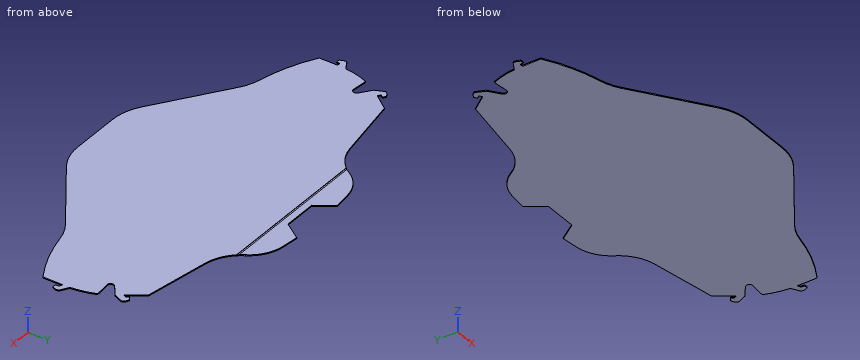
```python
from build123d import *

# Parameters (mm, degrees)
MAIN_SHAPE_DEPTH               = 0.6
TABS_DEPTH                     = 154.060061459
TABS_DEPTH_BACK                = 154.060061459
CHIN_GUARD_DEPTH               = 0.6
FILLET1_R                      = 30
QUICK_RELEASE_NOTCH_DEPTH      = 172.662513141
QUICK_RELEASE_NOTCH_DEPTH_BACK = 172.662513141
SKETCH8_W                      = 100
SKETCH8_H                      = 1
CUT_EXTRUDE3_DEPTH             = 0.2


with BuildPart() as part:
    # Sketch1 → Main Shape (new body)
    with BuildSketch(Plane.XY):
        with BuildLine():
            Line((-24, -91.764766734), (24, -91.764766734))
            Line((24, -91.764766734), (78.266232563, -84.05670244))
            ThreePointArc((78.266232563, -84.05670244), (97.655491519, -79.289252293), (115.711102551, -70.764766734))
            ThreePointArc((115.711102551, -70.764766734), (120.685143325, -65.658407438), (122.5, -58.764766734))
            ThreePointArc((122.5, -58.764766734), (120.227482046, -43.118277124), (113.597722286, -28.764766734))
            ThreePointArc((113.597722286, -28.764766734), (107.811505455, -22.955172168), (100.180351554, -19.955641477))
            Line((100.180351554, -19.955641477), (60.74391922, -13.264766734))
            ThreePointArc((60.74391922, -13.264766734), (50.804108255, -9.246591688), (43.461443341, -1.434367632))
            ThreePointArc((43.461443341, -1.434367632), (36.448172688, 5.805997675), (26.941855461, 9.15842781))
            Line((26.941855461, 9.15842781), (17, 10.235233266))
            Line((17, 10.235233266), (10, 0))
            Line((10, 0), (-10, 0))
            Line((-10, 0), (-17, 10.235233266))
            Line((-17, 10.235233266), (-26.941855461, 9.15842781))
            ThreePointArc((-26.941855461, 9.15842781), (-36.448172688, 5.805997675), (-43.461443341, -1.434367632))
            ThreePointArc((-43.461443341, -1.434367632), (-50.804108255, -9.246591688), (-60.74391922, -13.264766734))
            Line((-60.74391922, -13.264766734), (-100.180351554, -19.955641477))
            ThreePointArc((-100.180351554, -19.955641477), (-107.811505455, -22.955172168), (-113.597722286, -28.764766734))
            ThreePointArc((-113.597722286, -28.764766734), (-120.227482046, -43.118277124), (-122.5, -58.764766734))
            ThreePointArc((-122.5, -58.764766734), (-120.685143325, -65.658407438), (-115.711102551, -70.764766734))
            ThreePointArc((-115.711102551, -70.764766734), (-97.655491519, -79.289252293), (-78.266232563, -84.05670244))
            Line((-78.266232563, -84.05670244), (-24, -91.764766734))
        make_face()
    extrude(amount=MAIN_SHAPE_DEPTH)

    # Sketch2 → Tabs (cut, two sides: drawn at the far end of the back side and taken through both)
    with BuildSketch(Plane.XY.offset(0.6).offset(-TABS_DEPTH_BACK)):
        with BuildLine():
            Line((-121, -59.764766734), (-121, -57.764766734))
            Line((-121, -57.764766734), (-115.834995394, -54.767490128))
            ThreePointArc((-115.834995394, -54.767490128), (-113.511139955, -43.427720083), (-108.566362279, -32.961590783))
            Line((-108.566362279, -32.961590783), (-110.9, -27.464766734))
            Line((-110.9, -27.464766734), (-109.7, -25.864766734))
            Line((-109.7, -25.864766734), (-107.7, -24.864766734))
            Line((-107.7, -24.864766734), (-106.1, -26.064766734))
            Line((-106.1, -26.064766734), (-107.3, -27.664766734))
            Line((-107.3, -27.664766734), (-105.7, -28.864766734))
            Line((-105.7, -28.864766734), (-98.84870892, -19.729711961))
            Line((-98.84870892, -19.729711961), (-100.180351554, -19.955641477))
            ThreePointArc((-100.180351554, -19.955641477), (-107.811505455, -22.955172168), (-113.597722286, -28.764766734))
            ThreePointArc((-113.597722286, -28.764766734), (-120.227482046, -43.118277124), (-122.5, -58.764766734))
            ThreePointArc((-122.5, -58.764766734), (-120.767844146, -65.510135516), (-116, -70.586357152))
            Line((-116, -70.586357152), (-116, -59.764766734))
            Line((-116, -59.764766734), (-118, -59.764766734))
            Line((-118, -59.764766734), (-118, -61.764766734))
            Line((-118, -61.764766734), (-120, -61.764766734))
            Line((-120, -61.764766734), (-121, -59.764766734))
        make_face()
        with BuildLine():
            Line((109.7, -25.864766734), (110.9, -27.464766734))
            Line((110.9, -27.464766734), (108.566362279, -32.961590783))
            ThreePointArc((108.566362279, -32.961590783), (113.511139955, -43.427720083), (115.834995394, -54.767490128))
            Line((115.834995394, -54.767490128), (121, -57.764766734))
            Line((121, -57.764766734), (121, -59.764766734))
            Line((121, -59.764766734), (120, -61.764766734))
            Line((120, -61.764766734), (118, -61.764766734))
            Line((118, -61.764766734), (118, -59.764766734))
            Line((118, -59.764766734), (116, -58.764766734))
            Line((116, -58.764766734), (116, -70.586357152))
            ThreePointArc((116, -70.586357152), (120.767844146, -65.510135516), (122.5, -58.764766734))
            ThreePointArc((122.5, -58.764766734), (120.227482046, -43.118277124), (113.597722286, -28.764766734))
            ThreePointArc((113.597722286, -28.764766734), (107.811505455, -22.955172168), (100.180351554, -19.955641477))
            Line((100.180351554, -19.955641477), (98.84870892, -19.729711961))
            Line((98.84870892, -19.729711961), (105.979039493, -29.610311845))
            Line((105.979039493, -29.610311845), (106.979039493, -27.610311845))
            Line((106.979039493, -27.610311845), (105.920723622, -26.199224018))
            Line((105.920723622, -26.199224018), (107.7, -24.864766734))
            Line((107.7, -24.864766734), (109.7, -25.864766734))
        make_face()
    extrude(amount=TABS_DEPTH + TABS_DEPTH_BACK, mode=Mode.SUBTRACT)

    # Sketch5 → Chin guard (add)
    with BuildSketch(Plane.XY.offset(0.6)):
        Polygon((-78.266232563, -84.05670244), (-24, -121.764766734), (24, -121.764766734), (78.266232563, -84.05670244), (24, -91.764766734), (-24, -91.764766734), align=None)
    extrude(amount=-CHIN_GUARD_DEPTH)

    # Fillet1
    fillet1_edges = [part.edges().sort_by_distance(p)[0] for p in [
        (-24, -121.764766734, 0.3),
        (24, -121.764766734, 0.3),
        (78.266232563, -84.05670244, 0.3),
        (-78.266232563, -84.05670244, 0.3),
    ]]
    fillet(fillet1_edges, radius=FILLET1_R)

    # Sketch7 → Quick Release Notch (cut, two sides: drawn at the far end of the back side and taken through both)
    with BuildSketch(Plane.XY.offset(0.6).offset(-QUICK_RELEASE_NOTCH_DEPTH_BACK)):
        with BuildLine():
            Line((-103.483971257, -41.410990303), (-112.440490058, -40.52737785))
            ThreePointArc((-112.440490058, -40.52737785), (-110.669490914, -36.659449404), (-108.566362279, -32.961590783))
            Line((-108.566362279, -32.961590783), (-102.087612935, -37.820652791))
            ThreePointArc((-102.087612935, -37.820652791), (-101.423623928, -40.145597606), (-103.483971257, -41.410990303))
        make_face()
        with BuildLine():
            Line((108.566362279, -32.961590783), (102.087612935, -37.820652791))
            ThreePointArc((102.087612935, -37.820652791), (101.423623928, -40.145597606), (103.483971257, -41.410990303))
            Line((103.483971257, -41.410990303), (112.440490058, -40.52737785))
            ThreePointArc((112.440490058, -40.52737785), (110.669490914, -36.659449404), (108.566362279, -32.961590783))
        make_face()
    extrude(amount=QUICK_RELEASE_NOTCH_DEPTH + QUICK_RELEASE_NOTCH_DEPTH_BACK, mode=Mode.SUBTRACT)

    # Sketch8 → Cut-Extrude3 (cut)
    with BuildSketch(Plane.XY.offset(0.6)):
        with Locations((0, -4.5)):
            Rectangle(SKETCH8_W, SKETCH8_H)
    extrude(amount=-CUT_EXTRUDE3_DEPTH, mode=Mode.SUBTRACT)


solid = part.part
```
The listing builds one solid part. Answer for the finished solid, in the listing's coordinates (mm). Round coordinates to 2 decimals unless told otherwise and drop trailing zeros. Loops run counter-clockwise (first coordinate to the right, second up) from the corner with the lowest first, then second, coordinate; pieces in that order, holes last.
Q1. Section B-B, the plane x = 70.5 is taken. Determine the outline of the cut face in (y, z), then the cut area to 3 significant figures.
Q2. Given pin 1 Ø12 at (x, y) = (81.5, -92) entering from -Z, flat-ended and moving along its own axis, determine where the tip first touches the part or whether it passes through.
Q3. Section A-A, the plane y = -108.5 is taken. Determine the outline of the cut face in (x, z).
Q4. Find the intervals of material crossed by line 1 (X direction, y = -27, z = 0.2); line 2 (X direction, y = -25, z = 0.5); line 3 (Y direction, x = 4, z = 0.55), in increasing order.
Completed:
1. outline: (-89.45, 0) - (-14.92, 0) - (-14.92, 0.6) - (-89.45, 0.6) - close
1. area: 44.7 mm2
2. pin 1: passes through
3. outline: (-43.09, 0) - (43.09, 0) - (43.09, 0.6) - (-43.09, 0.6) - close
4. line 1: x = -110.55 to -106.8, -104.3 to 104.1, 106.52 to 110.55
4. line 2: x = -107.97 to -107.52, -102.8 to 102.65, 107.52 to 107.97
4. line 3: y = -121.76 to -5, -4 to 0
